from build123d import *

# Parameters (mm, degrees)
SKETCH1_W                                        = 123
SKETCH1_H                                        = 37
BOSS_EXTRUDE1_DEPTH                              = 6.5
CBORE_FOR_M4_HEX_HEAD_MACHINE_SCREW1_D           = 4.3
CBORE_FOR_M4_HEX_HEAD_MACHINE_SCREW1_CBORE_D     = 7
CBORE_FOR_M4_HEX_HEAD_MACHINE_SCREW1_CBORE_DEPTH = 3
SKETCH7_R                                        = 4
BOSS_EXTRUDE2_DEPTH                              = 25
SKETCH8_R                                        = 6
BOSS_EXTRUDE3_DEPTH                              = 7


with BuildPart() as part:
    # Sketch1 → Boss-Extrude1 (new body)
    with BuildSketch(Plane(origin=(0, 0, 0), x_dir=(1, 0, 0), z_dir=(0, 1, 0))):
        with Locations((61.5, 18.5)):
            Rectangle(SKETCH1_W, SKETCH1_H)
    extrude(amount=BOSS_EXTRUDE1_DEPTH)

    # CBORE for M4 Hex Head Machine Screw1 (through all)
    with Locations(Plane(origin=(0, 6.5, 0), x_dir=(1, 0, 0), z_dir=(0, 1, 0))):
        with Locations((5, 18.5), (118, 18.5)):
            CounterBoreHole(CBORE_FOR_M4_HEX_HEAD_MACHINE_SCREW1_D / 2, CBORE_FOR_M4_HEX_HEAD_MACHINE_SCREW1_CBORE_D / 2, CBORE_FOR_M4_HEX_HEAD_MACHINE_SCREW1_CBORE_DEPTH)

    # Sketch7 → Boss-Extrude2 (add)
    with BuildSketch(Plane(origin=(0, 6.5, 0), x_dir=(1, 0, 0), z_dir=(0, 1, 0))):
        with Locations((31, 18.5)):
            Circle(SKETCH7_R)
        with Locations((92, 18.5)):
            Circle(SKETCH7_R)
    extrude(amount=BOSS_EXTRUDE2_DEPTH)

    # Sketch8 → Boss-Extrude3 (add)
    with BuildSketch(Plane(origin=(0, 6.5, 0), x_dir=(1, 0, 0), z_dir=(0, 1, 0))):
        with Locations((31, 18.5)):
            Circle(SKETCH8_R)
        with Locations((92, 18.5)):
            Circle(SKETCH8_R)
    extrude(amount=BOSS_EXTRUDE3_DEPTH)


solid = part.part
Part model, mm, in its own coordinate system. A direction names the side the tool comes from. Give positions to 0.01 mm unless a question says otherwise; leave off trailing zeros. Loops run counter-clockwise (first coordinate to the right, second up) from the corner with the lowest first, then second, coordinate; pieces in that order, holes last. Notation, with made-up numbers: M 72,41 L 126,41 A31 ccw 126,66 Z; hole C 70,32 d10. An arc over 180 degrees is marked long. Put each result on its own line as item: value. Start each with the question number.
1) Saw through at A-A (x = 118). List the corners of the cut face in (y, z), then the cut area to 3 significant figures.
2) Saw through at B-B (y = 29.5). List the corners of the cut face in (x, z).
3) Saw through at C-C (x = 31). List the corners of the cut face in (y, z).
4) Flat gauge pins, fed straight in: pin 1 (5.5 mm diameter, centred on x = 5, z = -18.5, fed in from +Y); pin 2 (9 mm diameter, centred on x = 5, z = -18.5, fed in from +Y); pin 3 (10 mm diameter, centred on x = 38, y = 24.5, fed in from -Z). Where does each tip first touch, or does it go through?
5) Pull direction Z, two halves, no side cores. Call faces 3 (the cylindrical face through (121.34, 5.02, -19.55)), 4 (the flat face through (92, 31.5, -19)), 5 (the flat face through (61, 3, 0)): +Z half, -Z half, draft (parallel to the pull), parting line (faces both ways), or undercut.
6) 3-axis set-ups, long thin cutter, end or side, ignore diameter. For faces 1 (the flat face through (61, 0, -19)), 2 (the flat face through (7, 3.5, -20)): which of +Z, -Z, +X, -X, +Y, -Y reach the whole face in a straight line?
7) Saw through at D-D (z = -18.5). State how many separate pieces and enclosed holes the cut face has, then the cut area to 3 significant figures.
8) Probe probe 1 along X at (y, z) = (5.5, -18.5); probe 2 along X at (y, z) = (1.65, -18.5); probe 3 along Z at (x, y) = (5, 4). List the from-to ranges inside material, lowest first.
Numbers:
1. outline: M 0,-37 L 6.5,-37 L 6.5,-22 L 3.5,-22 L 3.5,-20.65 L 0,-20.65 Z; M 0,-16.35 L 3.5,-16.35 L 3.5,-15 L 6.5,-15 L 6.5,0 L 0,0 Z
1. area: 204 mm^2
2. outline: C 31,-18.5 d8; C 92,-18.5 d8
3. outline: M 0,-37 L 6.5,-37 L 6.5,-24.5 L 13.5,-24.5 L 13.5,-22.5 L 31.5,-22.5 L 31.5,-14.5 L 13.5,-14.5 L 13.5,-12.5 L 6.5,-12.5 L 6.5,0 L 0,0 Z
4. pin 1: y = 3.5
4. pin 2: y = 6.5
4. pin 3: z = -21.96
5. face 3: undercut
5. face 4: draft
5. face 5: +Z half
6. face 1: +Z, -Z, +X, -X, -Y
6. face 2: +Y
7. separate pieces: 3
7. enclosed holes: 0
7. area: 1,180 mm^2
8. probe 1: 0 to 1.5, 8.5 to 114.5, 121.5 to 123
8. probe 2: 0 to 2.85, 7.15 to 115.85, 120.15 to 123
8. probe 3: -37 to -22, -15 to 0
